from build123d import *

# Parameters (mm, degrees)
CYLINDER110_R     = 5.5
CYLINDER110_DEPTH = 60
CYLINDER109_R     = 8
CYLINDER109_DEPTH = 2.2


with BuildPart() as syringe_pusher_body:
    # Cylinder110 → Cylinder110 (new body)
    with BuildSketch(Plane.XY):
        Circle(CYLINDER110_R)
    extrude(amount=CYLINDER110_DEPTH)


with BuildPart() as syringe_pusher:
    # Cylinder109 → Cylinder109 (new body)
    with BuildSketch(Plane.XY.offset(60)):
        Circle(CYLINDER109_R)
    extrude(amount=CYLINDER109_DEPTH)

    # Fusion012: union syringe pusher body
    add(syringe_pusher_body.part)


with BuildPart() as syringe_pusher_1:
    # Fusion012 placement: moved
    add(syringe_pusher.part.moved(Location((0, 0, 27))))


solid = syringe_pusher_1.part
Part model, mm, in its own coordinate system. A direction names the side the tool comes from. Give positions to 0.01 mm unless a question says otherwise; leave off trailing zeros. Write each loop counter-clockwise with the first axis right and the second up, starting at its lowest first coordinate (ties: lowest second). Pieces come first, ordered by that corner, then holes.
1) Cut at A-A on y = 0. Write the cut outline in (x, z), then the cut area to 3 significant figures.
Resolved:
outline: (-8, 87) - (-5.5, 87) - (-5.5, 27) - (5.5, 27) - (5.5, 87) - (8, 87) - (8, 89.2) - (-8, 89.2) - close
area: 695 mm2
2) Which spindle directions (+Z, -Z, +X, -X, +Y, -Y) get a long thin tool onto all of the face, cutting with end or side? Do faces 1 (the face through (0, 0, 27)), 2 (the face through (-1.19, -5.37, 56.58)). Say none if no direction does.
Resolved:
face 1: -Z, +X, -X, +Y, -Y
face 2: -Z
3) Pin check, flat tips, straight feed: pin 1 (6 mm diameter, centred on x = -2.5, z = 82, fed in from +Y); pin 2 (6 mm diameter, centred on y = 2.5, z = 70.5, fed in from -X); pin 3 (3 mm diameter, centred on y = 2, z = 33.5, fed in from +X). Stop position of each tip, or through.
Resolved:
pin 1: stops at y = 5.5
pin 2: stops at x = -5.5
pin 3: stops at x = 5.48
4) Cut at D-D on y = -6.5. Write the cut outline in (x, z), then the cut area to 3 significant figures.
Resolved:
outline: (-4.66, 87) - (4.66, 87) - (4.66, 89.2) - (-4.66, 89.2) - close
area: 20.5 mm2
5) Cut at C-C on z = 67. Write the cut outline in (x, y).
Resolved:
outline: circle Ø11 at (0, 0)
6) Probe L1, parallel to Y at x = -0.25, z = 78.5; L2, parallel to Z at x = -5.5, y = -4.75. List the from-to ranges inside material, lowest first.
Resolved:
L1: y = -5.49 to 5.49
L2: z = 87 to 89.2
